Verification items for the finished model (mm, model axes). A direction names the side the tool comes from. Give positions to 0.01 mm unless a question says otherwise; leave off trailing zeros. Write each loop counter-clockwise with the first axis right and the second up, starting at its lowest first coordinate (ties: lowest second). Pieces come first, ordered by that corner, then holes. Notation, with made-up numbers: (-1.5, 13) - (39.5, 13) arc R12 ccw to (39.5, 20) - close; hole circle Ø2 at (-29.5, -29). An arc over 180 degrees is marked (long way). Answer as a JSON object with one key per item and string values. Group by question number.
Item 1: Sectioned sample at C-C, the plane y = 23. Record the boundary of the cut face in (x, z).
Item 2: Draft check along Z on faces 1 (the face through (1.091, -15.025, 15.38)), 2 (the face through (5.184, -2.194, 16.707)), 3 (the face through (-5.5, -13, 15)). Enter one of: +Z half, -Z half, draft (parallel to the pull), parting line (faces both ways), or undercut.
Item 3: Tool access check on faces 4 (the face through (3.1, -2, -25)), 5 (the face through (1.091, 15.38, 15.025)). Record the directions out of +Z, -Z, +X, -X, +Y, -Y that give a thin tool (end or side, any length) a straight path to the whole face; none if there is none.
Item 4: Go/stop test with flat-tipped pins: pin 1 (1 mm diameter, centred on x = 5.5, y = -13, fed in from +Z); pin 2 (9 mm diameter, centred on y = 0.5, z = -22.5, fed in from +X); pin 3 (2.5 mm diameter, centred on y = 1.5, z = 21.5, fed in from +X); pin 4 (2 mm diameter, centred on x = -3.5, z = 5.5, fed in from -Y). Record where each tip stops, or that it passes through.
Item 5: Sectioned sample at B-B, the plane y = 0. Count the separate pieces of the cut face and the enclosed holes in it, and give its area (3 significant figures).
Item 6: Scan lines: line 1 along Z through (x, y) = (-0.75, 0); line 2 along X through (y, z) = (10, 10.5); line 3 along X through (y, z) = (-7, 19.5). Record each from-to range of solid material in increasing order. Write a range as [from, to].
Item 7: Sectioned sample at A-A, the plane x = -3. Record the boundary of the cut face in (y, z).
Autodesk Inventor part; units mm, degrees
ref_plane "housing_to_dummy_XY" through (-7.5, 0, 0) normal (0, 0, 1) x (1, 0, 0)
ref_plane "housing_to_dummy_YZ" through (-7.5, 0, 0) normal (1, 0, 0) x (0, 1, 0)
ref_plane "housing_to_dummy_ZX" through (-7.5, 0, 0) normal (0, 1, 0) x (0, 0, 1)
sketch "Sketch_7" plane through (0, 0, 0) normal (0, 0, 1) x (1, 0, 0)
  line L0 (7.5, 0) -> (-7.5, 0)
  line L1 (-7.5, 0) -> (-7.5, 19)
  line L2 (-7.5, 19) -> (-5.8, 19)
  arc A0 (-5.8, 19) -> (-5.5, 19.3) centre (-5.8, 19.3) ccw
  line L3 (-5.5, 19.3) -> (-5.5, 28)
  line L4 (-5.5, 28) -> (7.5, 28)
  line L5 (7.5, 28) -> (7.5, 0)
  line L6 (7.5, 0) -> (-7.5, 0)
revolve "Revolution1" add sketch "Sketch_7" angle 360 about axis through (7.5, 0, 0) along (1, 0, 0)
sketch "Sketch_1" plane through (0, 0, 0) normal (0, 0, 1) x (1, 0, 0)
  line L0 (7.5, 0) -> (-7.5, 0)
  line L1 (-7.5, 0) -> (-7.5, 13)
  line L2 (-7.5, 13) -> (-5.5, 13)
  line L3 (-5.5, 13) -> (-5.5, 16)
  line L4 (-5.5, 16) -> (4.5, 16)
  line L5 (4.5, 16) -> (4.5, 16.85)
  line L6 (4.5, 16.85) -> (5.85, 16.85)
  line L7 (5.85, 16.85) -> (5.85, 16)
  line L8 (5.85, 16) -> (7.5, 16)
  line L9 (7.5, 16) -> (7.5, 0)
  line L10 (7.5, 0) -> (-7.5, 0)
revolve "Revolution2" cut sketch "Sketch_1" angle 360 about axis through (7.5, 0, 0) along (1, 0, 0)
sketch "Sketch_2" plane through (0, 0, 0) normal (0, 0, 1) x (1, 0, 0)
  line L0 (7.5, 23) -> (-5.5, 23)
  line L1 (-5.5, 23) -> (-5.5, 25.5)
  line L2 (-5.5, 25.5) -> (-5.067, 25.067)
  line L3 (-5.067, 25.067) -> (2.667, 25.067)
  line L4 (2.667, 25.067) -> (3.1, 25.5)
  line L5 (3.1, 25.5) -> (3.1, 27)
  line L6 (3.1, 27) -> (7.5, 27)
  line L7 (7.5, 27) -> (7.5, 23)
  line L8 (7.5, 23) -> (-5.5, 23)
revolve "Revolution3" cut sketch "Sketch_2" angle 360 about axis through (7.5, 23, 0) along (1, 0, 0)
thread "Thread1"
sketch "Sketch_4" plane through (7.5, 0, 0) normal (1, 0, 0) x (0, 0, -1)
  circle A0 centre (0, 0) radius 118.9529
  line L0 (-30.4056, 0) -> (0, -30.4056)
  line L1 (0, -30.4056) -> (30.4056, 0)
  line L2 (30.4056, 0) -> (0, 30.4056)
  line L3 (0, 30.4056) -> (-30.4056, 0)
extrude "Extrusion1" cut sketch "Sketch_4" against normal blind 15
pattern_linear "Rectangular Pattern1" count 2 spacing 32.5269 along (0, -0.7071, 0.7071) count 2 spacing 32.5269 along (0, -0.7071, -0.7071) of "Revolution3"
ref_plane "housing_to_dummy_XY" through (-7.5, 0, 0) normal (0, 0, 1) x (1, 0, 0)
ref_plane "housing_to_dummy_YZ" through (-7.5, 0, 0) normal (1, 0, 0) x (0, 1, 0)
ref_plane "housing_to_dummy_ZX" through (-7.5, 0, 0) normal (0, 1, 0) x (0, 0, 1)
ref_plane "to_bearings_XY" through (-5.5, 0, 0) normal (-1, 0, 0) x (0, 0, -1)
ref_plane "to_bearings_YZ" through (-5.5, 0, 0) normal (0, 0, -1) x (0, -1, 0)
ref_plane "to_bearings_ZX" through (-5.5, 0, 0) normal (0, -1, 0) x (-1, 0, 0)
ref_plane "to_rring_XY" through (4.5, 0, 0) normal (-1, 0, 0) x (0, 0, -1)
ref_plane "to_rring_YZ" through (4.5, 0, 0) normal (0, 0, -1) x (0, -1, 0)
ref_plane "to_rring_ZX" through (4.5, 0, 0) normal (0, -1, 0) x (-1, 0, 0)
properties part number "BGSRB6201ZZ_h"
Geometry check:
{
 "1": {"outline": "(-5.5, -7.41) - (7.5, -7.41) - (7.5, -4) - (3.1, -4) - (3.1, -2.5) - (2.67, -2.07) - (-5.07, -2.07) - (-5.5, -2.5) - close; (-5.5, 2.5) - (-5.07, 2.07) - (2.67, 2.07) - (3.1, 2.5) - (3.1, 4) - (7.5, 4) - (7.5, 7.41) - (-5.5, 7.41) - close"},
 "2": {"face 1": "+Z half", "face 2": "undercut", "face 3": "draft"},
 "3": {"face 4": "+X", "face 5": "+Z, +X, -X, +Y"},
 "4": {"pin 1": "z = 17.91", "pin 2": "x = 7.5", "pin 3": "x = 3.1", "pin 4": "y = -25.91"},
 "5": {"separate pieces": "4", "enclosed holes": "0", "area": "191 mm^2"},
 "6": {"line 1": "[-28, -25.07], [-20.93, -16], [16, 20.93], [25.07, 28]", "line 2": "[-7.5, -5.5]", "line 3": "[-5.5, 7.5]"},
 "7": {"outline": "(-27.89, -2.52) - (-2.52, -27.89) arc R28 ccw to (2.52, -27.89) - (27.89, -2.52) arc R28 ccw to (27.89, 2.52) - (2.52, 27.89) arc R28 ccw to (-2.52, 27.89) - (-27.89, 2.52) arc R28 ccw to start; hole circle Ø4.13 at (-23, 0); hole circle Ø32 at (0, 0); hole circle Ø4.13 at (0, -23); hole circle Ø4.13 at (0, 23); hole circle Ø4.13 at (23, 0)"}
}
